Design review of the part built by this model. Coordinates are the model's own, in mm. Face numbers are marked on the shaded views. A direction names the side the tool comes from. Round coordinates to 2 decimals unless told otherwise and drop trailing zeros. Order: outer loops, then holes, each group sorted by start corner. A loop starts at its lowest first (then second) coordinate and runs counter-clockwise, first axis right, second up. Notation, with made-up numbers: M 55,68 L 89,68 A15 ccw 89,73 Z; hole C 23.25,-30 d10. An arc over 180 degrees is marked long. Write item = value, one per line. Start each with the question number.
```python
from build123d import *

# Parameters (mm, degrees)
SKETCH_1_W          = 15
SKETCH_1_H          = 135
SKETCH_1_W_2        = 40
SKETCH_1_H_2        = 10
EXTRUDE_1_DEPTH     = 12
SKETCH_3_R          = 1.75
CUT_EXTRUDE_1_DEPTH = 128.157382798
FILLET_1_R          = 3
FILLET_2_R          = 5
FILLET_3_R          = 1
SKETCH_2_R          = 4.1
CUT_EXTRUDE_2_DEPTH = 5


with BuildPart() as part:
    # ｽｹｯﾁ1 → ﾎﾞｽ - 押し出し1 (new body)
    with BuildSketch(Plane.XY):
        Rectangle(SKETCH_1_W, SKETCH_1_H)
        with Locations((0, -62.5)):
            Rectangle(SKETCH_1_W_2, SKETCH_1_H_2)
    extrude(amount=EXTRUDE_1_DEPTH)

    # ｽｹｯﾁ3 → ｶｯﾄ - 押し出し1 (cut, through all)
    with BuildSketch(Plane(origin=(0, -57.5, 0), x_dir=(1, 0, 0), z_dir=(0, 1, 0))):
        with Locations(Location((-15, -6, 0), (0, 0, 270))):
            Circle(SKETCH_3_R)
        with Locations(Location((15, -6, 0), (0, 0, 270))):
            Circle(SKETCH_3_R)
    extrude(amount=-CUT_EXTRUDE_1_DEPTH, mode=Mode.SUBTRACT)

    # ﾌｨﾚｯﾄ1
    fillet_1_edges = [part.edges().sort_by_distance(p)[0] for p in [
        (-7.5, -57.5, 6),
        (7.5, -57.5, 6),
    ]]
    fillet(fillet_1_edges, radius=FILLET_1_R)

    # ﾌｨﾚｯﾄ2
    fillet_2_edges = [part.edges().sort_by_distance(p)[0] for p in [
        (7.5, 67.5, 6),
        (-7.5, 67.5, 6),
    ]]
    fillet(fillet_2_edges, radius=FILLET_2_R)

    # ﾌｨﾚｯﾄ3
    fillet_3_edges = [part.edges().sort_by_distance(p)[0] for p in [
        (20, -57.5, 6),
        (-20, -57.5, 6),
        (-15.25, -57.5, 12),
        (20, -62.5, 12),
        (-20, -62.5, 12),
        (-15.25, -57.5, 0),
        (20, -62.5, 0),
        (-20, -62.5, 0),
        (7.5, 4, 12),
        (7.5, 4, 0),
        (15.25, -57.5, 12),
        (15.25, -57.5, 0),
        (-7.5, 4, 12),
        (-7.5, 4, 0),
        (8.378679656, -56.621320344, 0),
        (8.378679656, -56.621320344, 12),
        (-8.378679656, -56.621320344, 0),
        (-8.378679656, -56.621320344, 12),
        (0, 67.5, 0),
        (0, 67.5, 12),
        (-6.035533906, 66.035533906, 0),
        (6.035533906, 66.035533906, 0),
        (-6.035533906, 66.035533906, 12),
        (6.035533906, 66.035533906, 12),
    ]]
    fillet(fillet_3_edges, radius=FILLET_3_R)

    # ｽｹｯﾁ2 → ｶｯﾄ - 押し出し2 (cut)
    with BuildSketch(Plane.XY.offset(12)):
        with Locations((0, 12.5)):
            Circle(SKETCH_2_R)
        with Locations((0, 62.5)):
            Circle(SKETCH_2_R)
    extrude(amount=-CUT_EXTRUDE_2_DEPTH, mode=Mode.SUBTRACT)


solid = part.part
```
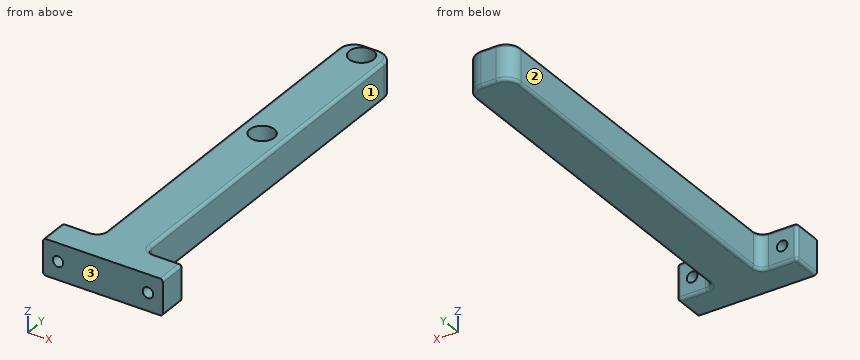
(1) Consider section D-D, the plane y = -5.5. Write out the cut boundary in (x, z), then the cut area to 3 significant figures.
(2) Consider section C-C, the plane z = 2.75. Write out the cut boundary in (x, y).
(3) For line 1 along Y through (x, z) = (0, 10.2); line 2 along X through (y, z) = (-63, 6); line 3 along X through (y, z) = (62.5, 10.9), list the stretches that pass through material, from the lowest coordinate up. Write a range as [from, to].
(4) Consider section A-A, the plane x = 15. Write out the cut boundary in (y, z), then the cut area to 3 significant figures.
(5) For the marked faces 1, 2 and 3, list the 3-axis set-ups (+Z, -Z, +X, -X, +Y, -Y) from which the entire face can be reached by the end or side of a thin tool; tool diameter is ignored.
(6) Consider section B-B, the plane y = 12.5. Write out the cut boundary in (x, z).
(7) Insertion check: pin 1 (4 mm diameter, centred on y = 21, z = 8.5, fed in from +X); pin 2 (4 mm diameter, centred on x = -15, z = 6, fed in from -Y); pin 3 (5 mm diameter, centred on x = 0, y = 62.5, fed in from +Z); pin 4 (2 mm diameter, centred on y = -5, z = 8.5, fed in from -X). Each pin has a flat end and moves straight along its axis. Give the tip position at first contact, or say it passes through.
Completed:
q1.outline = M -7.5,1 A1 ccw -6.5,0 L 6.5,0 A1 ccw 7.5,1 L 7.5,11 A1 ccw 6.5,12 L -6.5,12 A1 ccw -7.5,11 Z
q1.area = 179 mm2
q2.outline = M -20,-67.5 L 20,-67.5 L 20,-58.5 A1 ccw 19,-57.5 L 10.5,-57.5 A3 cw 7.5,-54.5 L 7.5,62.5 A5 ccw 2.5,67.5 L -2.5,67.5 A5 ccw -7.5,62.5 L -7.5,-54.5 A3 cw -10.5,-57.5 L -19,-57.5 A1 ccw -20,-58.5 Z
q3.line_1 = [-67.5, 8.4], [16.6, 58.4], [66.6, 67.5]
q3.line_2 = [-20, -16.75], [-13.25, 13.25], [16.75, 20]
q3.line_3 = [-7.5, -4.1], [4.1, 7.5]
q4.outline = M -67.5,0 L -58.5,0 A1 ccw -57.5,1 L -57.5,4.25 L -67.5,4.25 Z; M -67.5,7.75 L -57.5,7.75 L -57.5,11 A1 ccw -58.5,12 L -67.5,12 Z
q4.area = 84.6 mm2
q5.face_1 = +Z, -Z, +X, +Y
q5.face_2 = +Z, -Z, -X, +Y
q5.face_3 = +Z, -Z, +X, -X, -Y
q6.outline = M -7.5,1 A1 ccw -6.5,0 L 6.5,0 A1 ccw 7.5,1 L 7.5,11 A1 ccw 6.5,12 L 4.1,12 L 4.1,7 L -4.1,7 L -4.1,12 L -6.5,12 A1 ccw -7.5,11 Z
q7.pin_1 = 7.5
q7.pin_2 = -67.5
q7.pin_3 = 7
q7.pin_4 = -7.5
